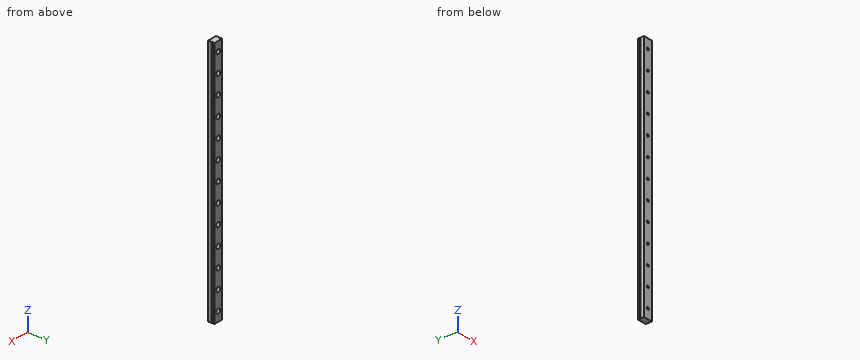
from build123d import *

# Parameters (mm, degrees)
BOSS_EXTRUDE1_DEPTH = 325
SKETCH3_R           = 1.5
CUT_EXTRUDE1_DEPTH  = 14
SKETCH4_R           = 3
CUT_EXTRUDE2_DEPTH  = 4.5
LPATTERN2_COUNT     = 14
LPATTERN2_PITCH     = 25


with BuildPart() as part:
    # Sketch1 → Boss-Extrude1 (new body)
    with BuildSketch(Plane.XY):
        with BuildLine():
            Line((-6, 1.5), (-5.4, 1.5))
            ThreePointArc((-5.4, 1.5), (-5.117157288, 1.382842712), (-5, 1.1))
            Line((-5, 1.1), (-5, 0.9))
            ThreePointArc((-5, 0.9), (-5.117157288, 0.617157288), (-5.4, 0.5))
            Line((-5.4, 0.5), (-6, 0.5))
            Line((-6, 0.5), (-6, -4))
            Line((-6, -4), (6, -4))
            Line((6, -4), (6, 0.5))
            Line((6, 0.5), (5.4, 0.5))
            ThreePointArc((5.4, 0.5), (5.117157288, 0.617157288), (5, 0.9))
            Line((5, 0.9), (5, 1.1))
            ThreePointArc((5, 1.1), (5.117157288, 1.382842712), (5.4, 1.5))
            Line((5.4, 1.5), (6, 1.5))
            Line((6, 1.5), (6, 3.5))
            Line((6, 3.5), (5.5, 4))
            Line((5.5, 4), (-5.5, 4))
            Line((-5.5, 4), (-6, 3.5))
            Line((-6, 3.5), (-6, 1.5))
        make_face()
    extrude(amount=BOSS_EXTRUDE1_DEPTH)

    # Sketch3 → Cut-Extrude1 (cut)
    with BuildSketch(Plane(origin=(0, 4, 0), x_dir=(1, 0, 0), z_dir=(0, 1, 0))):
        with Locations(Location((0, -312.5, 0), (0, 0, 270))):
            Circle(SKETCH3_R)
    cut_extrude1 = extrude(amount=-CUT_EXTRUDE1_DEPTH, mode=Mode.SUBTRACT)

    # Sketch4 → Cut-Extrude2 (cut)
    with BuildSketch(Plane(origin=(0, 4, 0), x_dir=(1, 0, 0), z_dir=(0, 1, 0))):
        with Locations(Location((0, -312.5, 0), (0, 0, 270))):
            Circle(SKETCH4_R)
    cut_extrude2 = extrude(amount=-CUT_EXTRUDE2_DEPTH, mode=Mode.SUBTRACT)

    # LPattern2: Cut-Extrude1, Cut-Extrude2 ×14
    with Locations(*[(0, 0, -i * LPATTERN2_PITCH) for i in range(1, LPATTERN2_COUNT)]):
        add(cut_extrude1, mode=Mode.SUBTRACT)
        add(cut_extrude2, mode=Mode.SUBTRACT)


solid = part.part
Verification items for the finished model (mm, model axes). Give positions to 0.01 mm unless a question says otherwise; leave off trailing zeros. Write each loop counter-clockwise with the first axis right and the second up, starting at its lowest first coordinate (ties: lowest second). Pieces come first, ordered by that corner, then holes.
(1) Cross-section at A-A (z = 193.5). Enter the section's corners in (x, y).
(2) Material ranges on line 1 (X direction, y = 1.05, z = 162.5); line 2 (Y direction, x = 5.5, z = 27); line 3 (X direction, y = 2.35, z = 112.5), recorded low to high.
(3) Gauge pin test, flat end, axial feed: pin 1 (5.5 mm diameter, centred on x = 0, z = 212.5, fed in from +Y). Record the tip position at first contact, or that the pin passes through.
Worked out:
1. outline: (-6, -4) - (6, -4) - (6, 0.5) - (5.4, 0.5) arc R0.4 cw to (5, 0.9) - (5, 1.1) arc R0.4 cw to (5.4, 1.5) - (6, 1.5) - (6, 3.5) - (5.5, 4) - (-5.5, 4) - (-6, 3.5) - (-6, 1.5) - (-5.4, 1.5) arc R0.4 cw to (-5, 1.1) - (-5, 0.9) arc R0.4 cw to (-5.4, 0.5) - (-6, 0.5) - close
2. line 1: x = -5 to -3, 3 to 5
2. line 2: y = -4 to 0.5, 1.5 to 4
2. line 3: x = -6 to -3, 3 to 6
3. pin 1: stops at y = -0.5
